```python
from build123d import *

# Parameters (mm, degrees)
FILLET1_R = 0.5


with BuildPart() as part:
    # Sketch1 → Revolve2 (revolve)
    with BuildSketch(Plane.XY):
        with BuildLine():
            Line((-6.5, 3.5), (-7.5, 3.5))
            Line((-7.5, 3.5), (-7.5, 4.5))
            Line((-7.5, 4.5), (-4.043760626, 4.5))
            ThreePointArc((-4.043760626, 4.5), (-2.459268184, 6.531675661), (0, 7.3))
            Line((0, 7.3), (0, -3.5))
            Line((0, -3.5), (-6.5, -3.5))
            Line((-6.5, -3.5), (-6.5, 3.5))
        make_face()
    revolve(axis=Axis((0, 7.3, 0), (0, -1, 0)))

    # Fillet1
    fillet1_edges = [part.edges().sort_by_distance(p)[0] for p in [
        (6.5, -3.5, 0),
    ]]
    fillet(fillet1_edges, radius=FILLET1_R)


solid = part.part
```
Could you check a few things on this model? Use its own coordinates, in mm. A direction names the side the tool comes from. Give positions to 0.01 mm unless a question says otherwise; leave off trailing zeros. Loops run counter-clockwise (first coordinate to the right, second up) from the corner with the lowest first, then second, coordinate; pieces in that order, holes last. Notation, with made-up numbers: (33.25, 83.25) - (65.25, 83.25) arc R19 ccw to (65.25, 97.25) - close; hole circle Ø8 at (88, -26.5). An arc over 180 degrees is marked (long way). Answer in a Markdown table with one row per item. Add a question column.
Q1. If we section it at C-C (y = 2.75): List the corners of the cut face in (x, z) for me.
Q2. If we section it at A-A (z = 0): List the corners of the cut face in (x, y) for me.
Q3. Please list where these lines run through material, in increasing order: L1, parallel to Y at x = -1.75, z = 6.5; L2, parallel to Y at x = -4.5, z = 1.25; L3, parallel to Z at x = -0.5, y = 3.75. Write a range as from..to.
Q4. For pin 1 (4 mm diameter, centred on y = 2.5, z = 4, fed in from +X); pin 2 (4 mm diameter, centred on y = 5.5, z = -5, fed in from -X); pin 3 (4 mm diameter, centred on x = -1, y = -2, fed in from +Z), each with a flat end and sliding along its axis, tell me the tip position at first contact or that it passes through.
Q5. Which directions (+Z, -Z, +X, -X, +Y, -Y) give clear straight access to the entire face, cutting with the end or side of a thin tool? Please do faces 1 (the face through (-3, 4.5, 3)), 2 (the face through (7.493, 4.007, -0.33)), 3 (the face through (-6, 3.5, -3)).
Q6. If we section it at B-B (x = 0): List the corners of the cut face in (y, z) for me, plus the area to 3 significant figures.
The answers:
| question | item | result |
|---|---|---|
| 1 | outline | circle Ø13 at (0, 0) |
| 2 | outline | (-7.5, 3.5) - (-6.5, 3.5) - (-6.5, -3) arc R0.5 ccw to (-6, -3.5) - (6, -3.5) arc R0.5 ccw to (6.5, -3) - (6.5, 3.5) - (7.5, 3.5) - (7.5, 4.5) - (4.04, 4.5) arc R4.32 ccw to (-4.04, 4.5) - (-7.5, 4.5) - close |
| 3 | L1 | y = 3.5..4.5 |
| 3 | L2 | y = -3.5..4.5 |
| 3 | L3 | z = -7.48..7.48 |
| 4 | pin 1 | stops at x = 7.15 |
| 4 | pin 2 | stops at x = -6.75 |
| 4 | pin 3 | stops at z = 6.5 |
| 5 | face 1 | +Y |
| 5 | face 2 | +Y, -Y |
| 5 | face 3 | -Y |
| 6 | outline | (-3.5, -6) arc R0.5 ccw to (-3, -6.5) - (3.5, -6.5) - (3.5, -7.5) - (4.5, -7.5) - (4.5, -4.04) arc R4.32 ccw to (4.5, 4.04) - (4.5, 7.5) - (3.5, 7.5) - (3.5, 6.5) - (-3, 6.5) arc R0.5 ccw to (-3.5, 6) - close |
| 6 | area | 122 mm^2 |
